from build123d import *

# Parameters (mm, degrees)
BOSS_EXTRUDE1_START = -300
SKETCH2_R           = 66
SKETCH2_R_2         = 58
BOSS_EXTRUDE1_DEPTH = 300
SKETCH3_R           = 132.244783432
CUT_EXTRUDE1_DEPTH  = 30


with BuildPart() as part:
    # Sketch1 → Revolve3 (revolve)
    with BuildSketch(Plane.XY, mode=Mode.PRIVATE) as revolve3_sk:
        with BuildLine():
            Line((76, -0.344450695), (76, 149.655549305))
            add(Edge.make_bspline(
                [(0.773326773, 400), (0.980987301, 399.685666805), (1.398059308, 399.052178662), (2.284541161, 397.700550841), (3.251241341, 396.211212549), (4.217116507, 394.710095548), (5.194582422, 393.178406868), (6.158529674, 391.654155139), (7.117841951, 390.123894266), (8.076303348, 388.581395306), (9.033719413, 387.026713906), (16.961041975, 374.037008419), (28.571782608, 353.014913091), (42.416505119, 323.258697721), (56.925249661, 282.331206246), (67.374040256, 242.08025425), (72.64853455, 209.220016816), (74.898010785, 183.923611768), (75.587535098, 169.173424136), (75.711753269, 165.955632222), (75.799260065, 163.208321649), (75.849799507, 161.393000412), (75.892883214, 159.587415565), (75.928787343, 157.784317211), (75.957511328, 155.967426666), (75.979054713, 154.18293971), (75.99341716, 152.40648291), (75.99880312, 150.790982345), (76, 150.032282914), (76, 149.655549305)],
                knots=[0.082616428, 0.082616428, 0.082616428, 0.082616428, 0.082616428, 0.088299706, 0.093982984, 0.099666263, 0.105349541, 0.111032819, 0.116716097, 0.122399375, 0.128082653, 0.133891142, 0.139699631, 0.313954311, 0.430124092, 0.546293874, 0.685697612, 0.836718331, 0.848335309, 0.865760775, 0.871569264, 0.877252541, 0.882935819, 0.888619096, 0.894302373, 0.899985651, 0.905668928, 0.911352205, 0.917035483, 0.917035483, 0.917035483, 0.917035483, 0.917035483], degree=4))
            Line((0.773326773, 400), (0.751990255, 381.399188372))
            add(Edge.make_bspline(
                [(0.751990255, 381.399188372), (0.873010956, 381.201299105), (3.80991255, 376.390848647), (12.106986141, 362.199887034), (29.393699031, 328.534275172), (48.723069726, 277.933780444), (60.486978792, 225.059949932), (64.620486576, 187.441870002), (65.581155817, 169.911010475), (65.839847213, 161.807957388), (65.916827257, 158.438692592), (65.954572398, 156.064661932), (65.971527827, 154.723430387), (65.981910919, 153.726401125), (65.989958451, 152.707134592), (65.995746725, 151.595575293), (65.999239242, 150.498770837), (66, 149.951992083), (66, 149.655549305)],
                knots=[0.132529105, 0.132529105, 0.132529105, 0.132529105, 0.134767619, 0.18691881, 0.291221192, 0.499825955, 0.708430719, 0.812733101, 0.864884292, 0.877922089, 0.890959887, 0.897478786, 0.900738235, 0.903997685, 0.907257134, 0.910516584, 0.913776033, 0.917035483, 0.917035483, 0.917035483, 0.917035483], degree=3))
            Line((66, 149.655549305), (66, -0.344450695))
            Line((66, -0.344450695), (76, -0.344450695))
        make_face()
    revolve(revolve3_sk.sketch.rotate(Axis((0, -198.817850362, 0), (0, -1, 0)), 270), axis=Axis((0, -198.817850362, 0), (0, -1, 0)))

    # Sketch2 → Boss-Extrude1 (add)
    with BuildSketch(Plane(origin=(0, 149.655549305, 0), x_dir=(1, 0, 0), z_dir=(0, 1, 0)).offset(BOSS_EXTRUDE1_START)):
        with Locations(Location((0, 0, 0), (0, 0, 270))):
            Circle(SKETCH2_R)
        with Locations(Location((0, 0, 0), (0, 0, 270))):
            Circle(SKETCH2_R_2, mode=Mode.SUBTRACT)
    extrude(amount=BOSS_EXTRUDE1_DEPTH)

    # Sketch3 → Cut-Extrude1 (cut)
    with BuildSketch(Plane(origin=(0, 400, 0), x_dir=(-1, 0, 0), z_dir=(0, -1, 0))):
        Circle(SKETCH3_R)
    extrude(amount=CUT_EXTRUDE1_DEPTH, mode=Mode.SUBTRACT)


solid = part.part
Work out the finished part from the listing and answer in its coordinate system (mm). A direction names the side the tool comes from. Round coordinates to 2 decimals unless told otherwise and drop trailing zeros. Write each loop counter-clockwise with the first axis right and the second up, starting at its lowest first coordinate (ties: lowest second). Pieces come first, ordered by that corner, then holes.
1) The mould has two halves that part along X. Classify faces 4 (the cylindrical face through (-22.21, -2.44, 53.58)), 5 (the cylindrical face through (-46.245, 75.706, 60.311)), 6 (the flat face through (-58.4, -150.344, -0.3)): pulls with the +X half, pulls with the -X half, needs draft (parallel to the pull), parting line crosses it, or undercut.
2) A cutting plane is placed at B-B (y = -28). Give the vertices of the cut face in (x, z).
3) Given pin 1 Ø8 at (x, y) = (54.5, 169) entering from +Z; pin 2 Ø1.5 at (y, z) = (74, -56.5) entering from -X; pin 3 Ø2 at (x, y) = (-40.5, 271) entering from -Z, each flat-ended and moving along its own axis, determine where each tip first touches the part or whether it passes through.
4) A tool of negligible diameter and unlimited length cuts with its end or side. For faces 1 (the flat face through (62.3, -0.344, -22.9)), 2 (the flat face through (-58.4, 149.656, -0.3)), 3 (the flat face through (0, 370, 8)), from which of +Z, -Z, +X, -X, +Y, -Y can it reach the whole face along a straight path? Write none if from no direction.
5) Straight lines are drawn through the part: line 1 (X direction, y = 28, z = 0); line 2 (X direction, y = -84.5, z = 2.5); line 3 (Z direction, x = -24.5, y = 268). For each, find the intervals that lie inside material, in ascending order.
6) A cutting plane is placed at A-A (y = 91). Give the vertices of the cut face in (x, z).
Completed:
1. face 4: undercut
1. face 5: parting line crosses it
1. face 6: needs draft
2. outline: circle Ø132 at (0, 0); hole circle Ø116 at (0, 0)
3. pin 1: stops at z = 56.25
3. pin 2: stops at x = -51.65
3. pin 3: stops at z = -44.56
4. face 1: -Y
4. face 2: none
4. face 3: +Z, -Z, +X, -X, +Y
5. line 1: x = -76 to -58, 58 to 76
5. line 2: x = -65.95 to -57.95, 57.95 to 65.95
5. line 3: z = -55.11 to -43.52, 43.52 to 55.11
6. outline: circle Ø152 at (0, 0); hole circle Ø116 at (0, 0)
